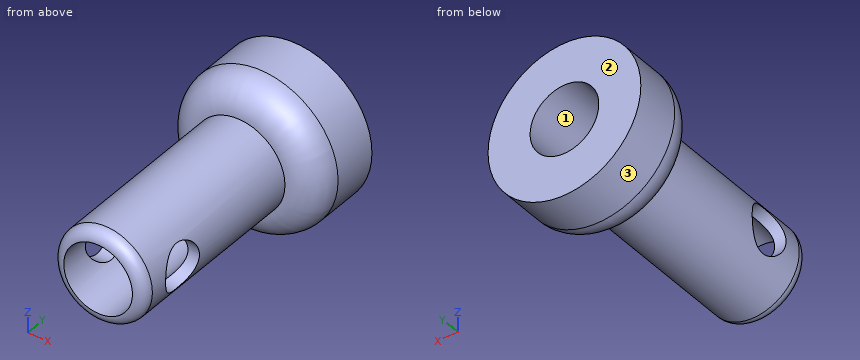
```python
from build123d import *

# Parameters (mm, degrees)
F0_R          = 50.8
F1_DEPTH      = 50.8
F2_R          = 20.32
F3_DEPTH      = 127
F4_R          = 7.62
F5_DEPTH      = 231.902
F6_R          = 15.24
F7_DEPTH      = 114.3
F7_DEPTH_BACK = 213.36


with BuildPart() as f1:
    # F0 (on Front) → F1 (new body)
    with BuildSketch(Plane.XZ):
        with Locations((-16.6321154684, 18.2440392673)):
            Circle(F0_R)
    extrude(amount=F1_DEPTH)

    # F2
    f2_edges = [f1.edges().sort_by_distance(p)[0] for p in [
        (-67.432115, -50.8, 18.244039),
    ]]
    fillet(f2_edges, radius=F2_R)

    # F3 (add): a face of the model
    f3_faces = [f1.faces().sort_by_distance(p)[0] for p in [
        (-16.6321154684, -50.8, 18.2440392673),
    ]]
    extrude(f3_faces, amount=F3_DEPTH)

    # F4
    f4_edges = [f1.edges().sort_by_distance(p)[0] for p in [
        (-47.112115, -177.8, 18.244039),
    ]]
    fillet(f4_edges, radius=F4_R)

    # F5 (cut): a face of the model
    f5_faces = [f1.faces().sort_by_distance(p)[0] for p in [
        (-16.6321154684, -177.8, 18.2440392673),
    ]]
    extrude(f5_faces, amount=-F5_DEPTH, mode=Mode.SUBTRACT)

    # F6 (on Right) → F7 (cut, two sides)
    with BuildSketch(Plane.YZ) as f7_sk:
        with Locations((-143.0514454842, 18.0790871382)):
            Circle(F6_R)
    extrude(amount=F7_DEPTH, mode=Mode.SUBTRACT)
    extrude(f7_sk.sketch, amount=-F7_DEPTH_BACK, mode=Mode.SUBTRACT)


solid = f1.part
```
Here's how the part is built. I have some questions about the finished solid (model axes, mm). Face numbers are marked on the shaded views. Coordinates: 2 decimals unless noted, no trailing zeros. Write each loop counter-clockwise with the first axis right and the second up, starting at its lowest first coordinate (ties: lowest second). Pieces come first, ordered by that corner, then holes. Notation, with made-up numbers: M 10.25,30 L 30.25,30 A22 ccw 30.25,67 Z; hole C 14.5,-39.75 d5. An arc over 180 degrees is marked long. Answer as CSV lines item,"result". Start each with the question number.
Q1. Suppose I cut it at A-A, the plane y = -155.5. List the corners of the cut face in (x, z) for me, then the cut area to 3 significant figures.
Q2. I need wall thicknesses on probe 1 along X at (y, z) = (-100, 37.5); probe 2 along Z at (x, y) = (-29.5, -41.5); probe 3 along Z at (x, y) = (-32, -168.5). Which ranges of each line are inside material? Lowest first, please. Write a range as [from, to].
Q3. Will these pins go through, and if not, where does the flat tip stop? pin 1 Ø5 at (x, y) = (1, -119.5) entering from +Z; pin 2 Ø1.5 at (y, z) = (-48, 7) entering from +X; pin 3 Ø6 at (y, z) = (-70, 22.5) entering from +X.
Q4. If we mould it in two halves opening along Z, with no side actions, what happens to the marked faces 1, 2 and 3? For each: pulls with the +Z half, pulls with the -Z half, needs draft (parallel to the pull), parting line crosses it, or undercut.
Q5. Suppose I cut it at C-C, the plane y = -18. List the corners of the cut face in (x, z) for me.
Q6. Suppose I cut it at B-B, the plane z = 24.5. State how many separate pieces and enclosed holes the cut face has, then the cut area to 3 significant figures.
Entries:
1,outline,"M -45.87,26.87 L -37.8,26.87 A22.86 cw 4.54,26.87 L 12.6,26.87 A30.48 ccw Z; M -45.77,9.29 A30.48 ccw 12.5,9.29 L 4.4,9.29 A22.86 cw -37.66,9.29 Z"
1,area,"1,000 mm²"
2,probe 1,"x = [-40.26, -28.95], [-4.31, 6.99]"
2,probe 2,"z = [-27.53, -0.65], [37.14, 64.02]"
2,probe 3,"z = [-8.08, 1.32], [35.17, 44.57]"
3,pin 1,"stops at z = 44.7"
3,pin 2,"stops at x = 23.81"
3,pin 3,"stops at x = 13.82"
4,face 1,"undercut"
4,face 2,"needs draft"
4,face 3,"parting line crosses it"
5,outline,"C -16.63,18.24 d101.6; hole C -16.63,18.24 d45.72"
6,separate pieces,"4"
6,enclosed holes,"0"
6,area,"4,240 mm²"
